Geometry check sheet. Reference: the model listing, model coordinates, mm. Face numbers are marked on the shaded views. A direction names the side the tool comes from. Coordinates: 2 decimals unless noted, no trailing zeros. Order: outer loops, then holes, each group sorted by start corner. A loop starts at its lowest first (then second) coordinate and runs counter-clockwise, first axis right, second up.
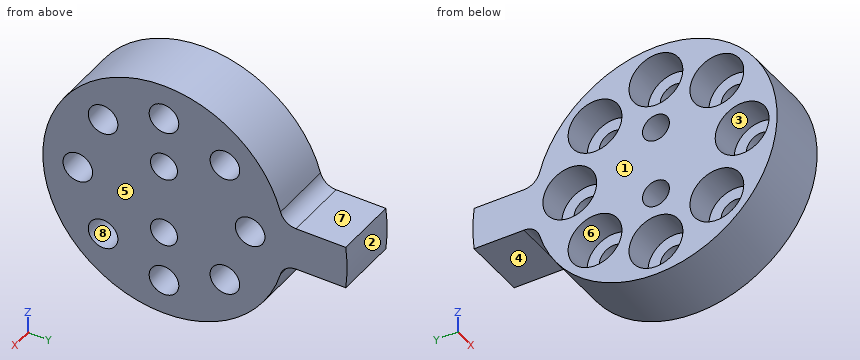
```python
from build123d import *

# Parameters (mm, degrees)
SKETCH_1_R                = 34
EXTRUDE_1_DEPTH           = 12
HOLE_WIZARD_1_D           = 5.5
HOLE_WIZARD_1_CBORE_D     = 10
HOLE_WIZARD_1_CBORE_DEPTH = 5.7
PATTERN_CIRCULAR_1_COUNT  = 8
SKETCH_4_OUTSIDE_W        = 89.382
SKETCH_4_OUTSIDE_H        = 89.382
CUT_EXTRUDE_2_DEPTH       = 50.558046773
HOLE_WIZARD_M6_1_D        = 5
FILLET_1_R                = 3


with BuildPart() as part:
    # 草图1 → 凸台-拉伸1 (new body)
    with BuildSketch(Plane(origin=(0, 0, 0), x_dir=(0, 0, -1), z_dir=(1, 0, 0))):
        Circle(SKETCH_1_R)
    extrude(amount=EXTRUDE_1_DEPTH)

    # 打孔尺寸根据内六角圆柱头螺钉的类型1 (through all)
    with Locations(Plane.ZY):
        with Locations((0, 16)):
            hole_wizard_1 = CounterBoreHole(HOLE_WIZARD_1_D / 2, HOLE_WIZARD_1_CBORE_D / 2, HOLE_WIZARD_1_CBORE_DEPTH)

    # 阵列(圆周)1: 打孔尺寸根据内六角圆柱头螺钉的类型1 ×8 about axis
    pattern_circular_1_axis = Axis((0, 0, 0), (1, 0, 0))
    for i in range(1, PATTERN_CIRCULAR_1_COUNT):
        add(hole_wizard_1.rotate(pattern_circular_1_axis, i * 360 / PATTERN_CIRCULAR_1_COUNT), mode=Mode.SUBTRACT)

    # 草图4 outside → 切除-拉伸2 (cut, through all)
    with BuildSketch(Plane.ZY):
        Rectangle(SKETCH_4_OUTSIDE_W, SKETCH_4_OUTSIDE_H)
        with BuildLine():
            Line((-4, 33.763886032), (-4, 22.141589825))
            ThreePointArc((-4, 22.141589825), (0, -22.5), (4, 22.141589825))
            Line((4, 22.141589825), (4, 33.763886032))
            ThreePointArc((4, 33.763886032), (0, 34), (-4, 33.763886032))
        make_face(mode=Mode.SUBTRACT)
    extrude(amount=-CUT_EXTRUDE_2_DEPTH, mode=Mode.SUBTRACT)

    # M6 螺纹孔1 (through all)
    with Locations(Plane.ZY):
        with Locations((6.5, 0), (-6.5, 0)):
            Hole(HOLE_WIZARD_M6_1_D / 2)

    # 圆角1
    fillet_1_edges = [part.edges().sort_by_distance(p)[0] for p in [
        (6, 22.141589825, 4),
        (6, 22.141589825, -4),
    ]]
    fillet(fillet_1_edges, radius=FILLET_1_R)


solid = part.part
```
Item 1: Sectioned sample at C-C (x = 2.5). Give the number of separate pieces and of enclosed holes in the cut face, and give its area (3 significant figures).
Item 2: Sectioned sample at B-B (y = -1.5). Record the cut outline in (x, z), and give its area (3 significant figures).
Item 3: Thickness scan on line 1 along Y through (x, z) = (7.75, 0); line 2 along Y through (x, z) = (4.5, -15.5); line 3 along Y through (x, z) = (8.75, 13). Record the ranges inside material, lowest first.
Item 4: Release check for a two-part mould opening along Y. For the marked faces 1, 2 and 3 record: pulls with the +Y half, pulls with the -Y half, needs draft (parallel to the pull), parting line crosses it, or undercut.
Item 5: Tool access check on the marked faces 4, 5, 6, 7 and 8. Record the directions out of +Z, -Z, +X, -X, +Y, -Y that give a thin tool (end or side, any length) a straight path to the whole face; none if there is none.
Item 6: Sectioned sample at A-A (z = 0). Record the cut outline in (x, y), and give its area (3 significant figures).
Item 7: Depth check by flat-ended pin: P1, Ø1.5, axis at y = 16.5, z = 15, coming from the -X side; P2, Ø4.5, axis at x = 8.5, y = 29, coming from the -Z side; P3, Ø8, axis at y = -0.5, z = -15.5, coming from the -X side; P4, Ø1, axis at x = 4, y = 9.5, coming from the -Z side. Enter the tip coordinate at first touch or a pass-through.
Geometry check:
1. separate pieces: 1
1. enclosed holes: 10
1. area: 1,020 mm2
2. outline: (0, -22.45) - (12, -22.45) - (12, -18.3) - (5.7, -18.3) - (5.7, -20.77) - (0, -20.77) - close; (0, -11.23) - (5.7, -11.23) - (5.7, -13.7) - (12, -13.7) - (12, -8.5) - (0, -8.5) - close; (0, -4.5) - (12, -4.5) - (12, 4.5) - (0, 4.5) - close; (0, 8.5) - (12, 8.5) - (12, 13.7) - (5.7, 13.7) - (5.7, 11.23) - (0, 11.23) - close; (0, 20.77) - (5.7, 20.77) - (5.7, 18.3) - (12, 18.3) - (12, 22.45) - (0, 22.45) - close
2. area: 276 mm2
3. line 1: y = -22.5 to -18.75, -13.25 to 13.25, 18.75 to 34
3. line 2: y = -16.31 to -14.05, -8.58 to -4.97, 4.97 to 8.58, 14.05 to 16.31
3. line 3: y = -18.36 to -13.49, -9.14 to 9.14, 13.49 to 18.36
4. face 1: needs draft
4. face 2: pulls with the +Y half
4. face 3: undercut
5. face 4: -Z, +X, -X, +Y
5. face 5: +Z, -Z, +X, +Y, -Y
5. face 6: -X
5. face 7: +Z, +X, -X, +Y
5. face 8: +X, -X
6. outline: (0, -22.5) - (12, -22.5) - (12, -18.75) - (5.7, -18.75) - (5.7, -21) - (0, -21) - close; (0, -11) - (5.7, -11) - (5.7, -13.25) - (12, -13.25) - (12, 13.25) - (5.7, 13.25) - (5.7, 11) - (0, 11) - close; (0, 21) - (5.7, 21) - (5.7, 18.75) - (12, 18.75) - (12, 34) - (0, 34) - close
6. area: 495 mm2
7. P1: stops at x = 0
7. P2: stops at z = -4
7. P3: stops at x = 5.7
7. P4: stops at z = -20.62
